Check sheet for the modelled part. Datum: model origin and axes. Units: mm. A direction names the side the tool comes from. Coordinates: 2 decimals unless noted, no trailing zeros. Loops run counter-clockwise (first coordinate to the right, second up) from the corner with the lowest first, then second, coordinate; pieces in that order, holes last. Notation, with made-up numbers: M 22.5,60 L 57.5,60 A31 cw 57.5,89 Z; hole C -18,36 d11. An arc over 180 degrees is marked long. Answer in a Markdown table with one row per item. Add a question column.
```python
from build123d import *

# Parameters (mm, degrees)
F2_R      = 3.175
F3_DEPTH  = 38.1
F4_R      = 3.175
F5_DEPTH  = 38.1
F7_DEPTH  = 6.35
F8_SIZE   = 1.905
F9_R      = 3.175
F10_DEPTH = 9.525


# Not quite as in the source:
# - a feature names something its author has since deleted; it is built from what else it names


with BuildPart() as f1:
    # F0 (on Front) → F1 (revolve)
    with BuildSketch(Plane.XZ):
        Polygon((41.9862, 25.4), (41.9862, 0), (48.3362, 0), (48.3362, 25.527), (48.3362, 38.1), (45.1612, 38.1), (45.1612, 34.925), (38.8112, 34.925), (38.8112, 31.3944), (35.2806, 31.3944), (35.2806, 34.925), (28.9306, 34.925), (28.9306, 32.385), (22.5806, 32.385), (22.5806, 34.925), (16.2306, 34.925), (16.2306, 31.3944), (12.7, 31.3944), (12.7, 34.925), (0, 34.925), (0, 25.4), (5.08, 25.4), (5.08, 28.9306), (8.6106, 28.9306), (8.6106, 25.4), align=None)
    revolve(axis=Axis((-0.433858484, 0, 0), (1, 0, 0)))

    # F2 (on Front) → F3 (cut, symmetric)
    with BuildSketch(Plane.XZ):
        with Locations((25.9468089789, 0)):
            Circle(F2_R)
    extrude(amount=F3_DEPTH, both=True, mode=Mode.SUBTRACT)

    # F4 (on Top) → F5 (cut, symmetric)
    with BuildSketch(Plane.XY):
        with Locations((26.0544512421, 0)):
            Circle(F4_R)
    extrude(amount=F5_DEPTH, both=True, mode=Mode.SUBTRACT)

    # F7 (add): a face of the model
    f7_faces = [f1.faces().sort_by_distance(p)[0] for p in [
        (48.3362, 0, 0),
    ]]
    extrude(f7_faces, amount=F7_DEPTH)

    # F8
    f8_edges = [f1.edges().sort_by_distance(p)[0] for p in [
        (0, 0, -34.925),
    ]]
    chamfer(f8_edges, length=F8_SIZE)

    # F9 (on face) → F10 (cut)
    with BuildSketch(Plane.YZ.offset(54.6862)):
        with Locations((13.4703841816, 13.4703841816)):
            Circle(F9_R)
        with Locations((13.4703841816, -13.4703841816)):
            Circle(F9_R)
        with Locations((-13.4703841816, -13.4703841816)):
            Circle(F9_R)
        with Locations((-13.4703841816, 13.4703841816)):
            Circle(F9_R)
    extrude(amount=-F10_DEPTH, mode=Mode.SUBTRACT)


solid = f1.part
```
Q1. Cross-section at A-A (x = 25.5). Record the cut outline in (y, z) (3 decimals).
Q2. Thickness scan on L1, parallel to Z at x = 7, y = 0 (3 decimals); L2, parallel to X at y = 20.5, z = -20; L3, parallel to X at y = 0, z = 31.75. Record the ranges inside material, lowest first.
Q3. Cross-section at B-B (y = 0). Count the separate pieces of the cut face and the enclosed holes in it, plus the area to 3 significant figures.
Q4. Access from +Z, -Z, +X, -X, +Y, -Y to the whole of each face (thin tool, end or side, straight path). Record for faces 1 (the face through (25.532, -7.629, 24.227)), 2 (the face through (37.021, -9.43, 29.945)), 3 (the face through (28.931, -23.2, -23.1)).
Q5. Mould release check, pull along Y, two halves, no side actions. Record for faces 4 (the face through (41.986, 0, 0)), 5 (the face through (0, 19.4, 17)), 6 (the face through (41.942, 21.251, -27.715)): released by +Y, released by -Y, zero draft, split by the parting line, or undercut.
Q6. Go/stop test with flat-tipped pins: pin 1 (6 mm diameter, centred on x = 22.5, z = 20, fed in from -Y); pin 2 (5 mm diameter, centred on y = -13.47, z = -13.47, fed in from -X); pin 3 (5 mm diameter, centred on x = 7, y = 24.5, fed in from +Z). Record where each tip stops, or that it passes through.
Answer key:
| question | item | result |
|---|---|---|
| 1 | outline | M -32.232,-3.143 A32.385 ccw -3.126,-32.234 L -3.126,-25.207 A25.4 cw -25.205,-3.143 Z; M -32.232,3.143 L -25.205,3.143 A25.4 cw -3.126,25.207 L -3.126,32.234 A32.385 ccw Z; M 3.126,-32.234 A32.385 ccw 32.232,-3.143 L 25.205,-3.143 A25.4 cw 3.126,-25.207 Z; M 3.126,25.207 A25.4 cw 25.205,3.143 L 32.232,3.143 A32.385 ccw 3.126,32.234 Z |
| 2 | L1 | -34.925 to -28.931, 28.931 to 34.925 |
| 2 | L2 | 0 to 5.08, 8.61 to 54.69 |
| 2 | L3 | 0 to 12.7, 16.23 to 22.88, 29.23 to 35.28, 38.81 to 54.69 |
| 3 | separate pieces | 3 |
| 3 | enclosed holes | 0 |
| 3 | area | 1,550 mm^2 |
| 4 | face 1 | -X |
| 4 | face 2 | none |
| 4 | face 3 | -Z, -Y |
| 5 | face 4 | undercut |
| 5 | face 5 | zero draft |
| 5 | face 6 | split by the parting line |
| 6 | pin 1 | y = -30.51 |
| 6 | pin 2 | x = 41.99 |
| 6 | pin 3 | z = 27.12 |
